from build123d import *


with BuildPart() as part:
    # Sketch1 → Revolve1 (revolve)
    with BuildSketch(Plane.XY, mode=Mode.PRIVATE) as revolve1_sk:
        with BuildLine():
            Line((0, 0), (-4, 0))
            Line((-4, 0), (-4, 7))
            Line((-4, 7), (-5, 7))
            Line((-5, 7), (-5, 19))
            Line((-5, 19), (-7.5, 19))
            Line((-7.5, 19), (-7.5, 21))
            ThreePointArc((-7.5, 21), (-7.207106781, 21.707106781), (-6.5, 22))
            Line((-6.5, 22), (0, 22))
            Line((0, 22), (0, 0))
        make_face()
    revolve(revolve1_sk.sketch.rotate(Axis((0, 22, 0), (0, -1, 0)), 270), axis=Axis((0, 22, 0), (0, -1, 0)))


solid = part.part
Verification items for the finished model (mm, model axes). Coordinates: 2 decimals unless noted, no trailing zeros. Order: outer loops, then holes, each group sorted by start corner. A loop starts at its lowest first (then second) coordinate and runs counter-clockwise, first axis right, second up.
1. Release check for a two-part mould opening along Y. For faces 1 (the face through (-0.33, 20.014, -7.493)), 2 (the face through (0, 0, 0)), 3 (the face through (0, 22, 0)) record: +Y half, -Y half, draft (parallel to the pull), parting line (faces both ways), or undercut.
Results found:
face 1: draft
face 2: -Y half
face 3: +Y half
2. Sectioned sample at A-A, the plane x = 0. Record the cut outline in (y, z), and give its area (3 significant figures).
Results found:
outline: (0, -4) - (7, -4) - (7, -5) - (19, -5) - (19, -7.5) - (21, -7.5) arc R1 ccw to (22, -6.5) - (22, 6.5) arc R1 ccw to (21, 7.5) - (19, 7.5) - (19, 5) - (7, 5) - (7, 4) - (0, 4) - close
area: 221 mm2
3. Scan lines: line 1 (Y direction, x = -5.75, z = 3); line 2 (X direction, y = 9, z = -0.25); line 3 (Y direction, x = -3, z = -3.25). Record each from-to range of solid material in increasing order.
Results found:
line 1: y = 19 to 22
line 2: x = -4.99 to 4.99
line 3: y = 7 to 22
4. Sectioned sample at B-B, the plane z = 0. Record the cut outline in (x, y), and give its area (3 significant figures).
Results found:
outline: (-7.5, 19) - (-5, 19) - (-5, 7) - (-4, 7) - (-4, 0) - (4, 0) - (4, 7) - (5, 7) - (5, 19) - (7.5, 19) - (7.5, 21) arc R1 ccw to (6.5, 22) - (-6.5, 22) arc R1 ccw to (-7.5, 21) - close
area: 221 mm2
5. Go/stop test with flat-tipped pins: pin 1 Ø4 at (y, z) = (3.5, 0.5) entering from +X; pin 2 Ø2 at (y, z) = (15.5, -3) entering from -X; pin 3 Ø8 at (y, z) = (10, -5.5) entering from +X; pin 4 Ø8 at (x, z) = (1.5, 1) entering from -Y. Record where each tip stops, or that it passes through.
Results found:
pin 1: stops at x = 4
pin 2: stops at x = -4.58
pin 3: stops at x = 4.77
pin 4: stops at y = 0
6. Sectioned sample at D-D, the plane y = 10.5. Record the cut outline in (x, z), and give its area (3 significant figures).
Results found:
outline: circle Ø10 at (0, 0)
area: 78.5 mm2
7. Sectioned sample at C-C, the plane y = 19.75. Record the cut outline in (x, z), and give its area (3 significant figures).
Results found:
outline: circle Ø15 at (0, 0)
area: 177 mm2
